Could you check a few things on this model? Use its own coordinates, in mm. A direction names the side the tool comes from. Round coordinates to 2 decimals unless told otherwise and drop trailing zeros. Write each loop counter-clockwise with the first axis right and the second up, starting at its lowest first coordinate (ties: lowest second). Pieces come first, ordered by that corner, then holes.
Autodesk Inventor part; units mm, degrees
ref_plane "YZ Plane" through (0, 0, 0) normal (1, 0, 0) x (0, 1, 0)
ref_plane "XZ Plane" through (0, 0, 0) normal (0, 1, 0) x (-1, 0, 0)
ref_plane "XY Plane" through (0, 0, 0) normal (0, 0, 1) x (1, 0, 0)
sketch "Sketch1" plane through (0, 0, 0) normal (0, 1, 0) x (-1, 0, 0)
  circle A0 centre (0, 0) radius 57
  circle A1 centre (0, 0) radius 50
  line L0 (0, -92.0258) -> (0, 121.5043)
  line L1 (123.2816, 0) -> (-123.2816, 0)
  line L2 (-50, 2) -> (50, 2)
  line L3 (50, 2) -> (50, -2)
  line L4 (50, -2) -> (-50, -2)
  line L5 (-50, -2) -> (-50, 2)
  line L6 (-50, 2) -> (50, -2) construction
  line L7 (50, 2) -> (-50, -2) construction
  line L8 (2, 50) -> (-2, 50)
  line L9 (-2, 50) -> (-2, -50)
  line L10 (-2, -50) -> (2, -50)
  line L11 (2, -50) -> (2, 50)
  line L12 (2, 50) -> (-2, -50) construction
  line L13 (-2, 50) -> (2, -50) construction
  line L14 (18.5, 91) -> (-18.5, 91)
  line L15 (-18.5, 91) -> (-18.5, 50)
  line L16 (-18.5, 50) -> (18.5, 50)
  line L17 (18.5, 50) -> (18.5, 91)
  line L18 (0, 91) -> (0, 50) construction
  line L19 (18.5, 60) -> (-18.5, 60)
  line L20 (-44.3013, -23.2679) -> (-42.3013, -26.7321)
  line L21 (-34.0513, -41.0215) -> (-52.5513, -8.9785)
  line L22 (-61.2115, -13.9785) -> (-42.7115, -46.0215)
  line L23 (-69.5583, -61.5215) -> (-34.0513, -41.0215)
  line L24 (-52.5513, -8.9785) -> (-88.0583, -29.4785)
  line L25 (-78.8083, -45.5) -> (-43.3013, -25) construction
  line L26 (-88.0583, -29.4785) -> (-69.5583, -61.5215)
  line L27 (42.3013, -26.7321) -> (44.3013, -23.2679)
  line L28 (52.5513, -8.9785) -> (34.0513, -41.0215)
  line L29 (42.7115, -46.0215) -> (61.2115, -13.9785)
  line L30 (88.0583, -29.4785) -> (52.5513, -8.9785)
  line L31 (34.0513, -41.0215) -> (69.5583, -61.5215)
  line L32 (78.8083, -45.5) -> (43.3013, -25) construction
  line L33 (69.5583, -61.5215) -> (88.0583, -29.4785)
  point P0 (2, -49.96)
  point P1 (2, -2)
  point P2 (49.96, -2)
  point P3 (-2, 49.96)
  point P4 (-2, 2)
  point P5 (-49.96, 2)
  point P6 (-2, -49.96)
  point P7 (-49.96, -2)
  point P8 (-2, -2)
  point P9 (-18.5, 53.9143)
  point P10 (-55.9411, -10.9357)
  point P11 (-37.4411, -42.9786)
  point P12 (37.4411, -42.9786)
  point P13 (55.9411, -10.9357)
  point P14 (18.5, 53.9143)
  point P15 (2, 49.96)
  point P16 (49.96, 2)
  point P17 (2, 2)
  dimension "d0" = 114
  dimension "d1" = 100
  dimension "d6" = 100
  dimension "d7" = 4
  dimension "d8" = 4
  dimension "d9" = 100
  dimension "d10" = 37
  dimension "d14" = 60
  dimension "d15" = 31
  dimension "d18" = 360
extrude "Extrusion1" add sketch "Sketch1" along normal blind 5 contours L1 L3 L2 A1 L11 L16 L17 A0 | A0 L30 L28 L27 A1 L4 L3 L1 | L17 L16 L8 L0 A0 | A0 L0 L19 L17 | L30 L29 L31 A0 | A0 L31 L28 L27 L30 | L1 L11 L2 A1 | L3 L4 A1 | A1 L4 L11 L1 | A1 L2 L3 | L0 L8 L16 L15 A0 | A0 L15 L19 L0 | L19 L0 L14 L17 | A0 L0 L10 L11 A1 L27 L28 L31 | L30 L33 L31 L29 | L11 L4 L0 L1 | L1 L0 L2 L11 | L15 L16 L9 A1 L2 L5 L1 A0 | L8 L11 A1 | L0 L2 L9 A1 | A1 L11 L2 L0 | A1 L9 L8 | L19 L15 L14 L0 | A0 L23 L21 L20 A1 L9 L10 L0 | L11 A1 L0 L4 | L1 L9 L2 L0 | L0 L4 L9 L1 | L1 L5 L4 A1 L20 L21 L24 A0 | L23 L22 L24 A0 | A0 L24 L21 L20 L23 | L10 L9 A1 | A1 L9 L4 L0 | A1 L11 L10 | L9 L4 A1 L1 | L1 A1 L2 L9 | L5 L2 A1 | A1 L4 L5 | L23 L26 L24 L22
sketch "Sketch2" plane through (0, 5, 0) normal (0, 1, 0) x (1, 0, 0)
  line L0 (-18.5, -53.9143) -> (-18.5, -91)
  line L1 (18.5, -91) -> (18.5, -53.9143)
  line L2 (-18.5, -91) -> (18.5, -91)
  line L3 (18.5, -91) -> (18.5, -60)
  line L4 (18.5, -60) -> (-18.5, -60)
  line L5 (-18.5, -60) -> (-18.5, -91)
  line L6 (-17, -61.5) -> (17, -61.5)
  line L7 (17, -61.5) -> (17, -89.5)
  line L8 (17, -89.5) -> (-17, -89.5)
  line L9 (-17, -89.5) -> (-17, -61.5)
  line L10 (88.0583, 29.4785) -> (69.5583, 61.5215)
  line L11 (69.5583, 61.5215) -> (42.7115, 46.0215)
  line L12 (42.7115, 46.0215) -> (61.2115, 13.9785)
  line L13 (61.2115, 13.9785) -> (88.0583, 29.4785)
  line L14 (61.7606, 16.0276) -> (44.7606, 45.4724)
  line L15 (44.7606, 45.4724) -> (69.0093, 59.4724)
  line L16 (69.0093, 59.4724) -> (86.0093, 30.0276)
  line L17 (86.0093, 30.0276) -> (61.7606, 16.0276)
  line L18 (-69.5583, 61.5215) -> (-88.0583, 29.4785)
  line L19 (-88.0583, 29.4785) -> (-61.2115, 13.9785)
  line L20 (-61.2115, 13.9785) -> (-42.7115, 46.0215)
  line L21 (-42.7115, 46.0215) -> (-69.5583, 61.5215)
  line L22 (-44.7606, 45.4724) -> (-61.7606, 16.0276)
  line L23 (-61.7606, 16.0276) -> (-86.0093, 30.0276)
  line L24 (-86.0093, 30.0276) -> (-69.0093, 59.4724)
  line L25 (-69.0093, 59.4724) -> (-44.7606, 45.4724)
  point P0 (0, 0)
  dimension "d22" = 31
  dimension "d23" = 1.5
  dimension "d26" = 360
extrude "Extrusion2" add sketch "Sketch2" along normal blind 46 contours L4 L1 L2 L0
sketch "Sketch4" plane through (-18.5, 0, 91) normal (0, 0, 1) x (1, 0, 0)
  line L0 (0, 51) -> (37, 51) construction
  line L1 (12.5, 51) -> (24.5, 51)
  line L2 (24.5, 51) -> (24.5, 10)
  line L3 (24.5, 10) -> (12.5, 10)
  line L4 (12.5, 10) -> (12.5, 51)
  line L5 (1.5, 5) -> (35.5, 5) construction
  line L6 (18.5, -10.2) -> (18.5, 61.2) construction
  circle A0 centre (18.5, 16) radius 6
  point P0 (18.5, 0)
  point P1 (12.5, 16)
  point P2 (24.5, 16)
  dimension "d36" = 12
  dimension "d37" = 5
  dimension "d38" = 6
extrude "Extrusion3" cut sketch "Sketch4" against normal up to next contours L1 L2 A0 L4 | A0
pattern_circular "Circular Pattern1" count 3 over 360 about axis through (0, -10, 0) along (0, 1, 0) of "Extrusion2", "Extrusion3"
sketch "Sketch5" plane through (0, 5, 0) normal (0, 1, 0) x (1, 0, 0)
  line L0 (-2, -21.5) -> (2, -21.5)
  line L1 (2, -21.5) -> (2, -17.5)
  line L2 (2, -17.5) -> (-2, -17.5)
  line L3 (-2, -17.5) -> (-2, -21.5)
  line L4 (-2, -2) -> (-2, -49.96) construction
  line L5 (2, -49.96) -> (2, -2) construction
  line L6 (-123.2816, 0) -> (123.2816, 0) construction
  line L7 (-2, 21.5) -> (2, 21.5)
  line L8 (2, 21.5) -> (2, 17.5)
  line L9 (2, 17.5) -> (-2, 17.5)
  line L10 (-2, 17.5) -> (-2, 21.5)
  arc A0 (-49.96, -2) -> (-2, -49.96) centre (0, 0) ccw construction
  arc A1 (-2, 49.96) -> (-49.96, 2) centre (0, 0) ccw construction
  circle A2 centre (0, 0) radius 50 construction
  line L11 (-54, 6) -> (-50, 6)
  line L12 (-50, 6) -> (-50, -6)
  line L13 (-50, -6) -> (-54, -6)
  line L14 (-54, -6) -> (-54, 6)
  line L15 (-54, 0) -> (-50, 0) construction
  line L16 (0, 92.0258) -> (0, -121.5043) construction
  line L17 (54, 6) -> (50, 6)
  line L18 (50, 6) -> (50, -6)
  line L19 (50, -6) -> (54, -6)
  line L20 (54, -6) -> (54, 6)
  line L21 (54, 0) -> (50, 0) construction
  point P0 (49.96, -2)
  point P1 (49.96, 2)
  dimension "d41" = 17.5
  dimension "d42" = 4
  dimension "d43" = 12
extrude "Extrusion4" add sketch "Sketch5" along normal blind 10
equation "\"d38\" = 0.5 * d36"
properties part number "bottom"
Q1. We'd pull the mould along X, two halves only. Please class faces 1 (the flat face through (52, 10, 6)), 2 (the flat face through (-74.823, 27.678, -21.837)), 3 (the flat face through (71.775, 2.465, -20.077)), 4 (the flat face through (-26, 2, -2)): pulls with the +X half, pulls with the -X half, needs draft (parallel to the pull), parting line crosses it, or undercut.
Q2. On a 3-axis mill with a long thin cutter (end or side, diameter ignored), from which of +Z, -Z, +X, -X, +Y, -Y can I reach the whole of each face in a straight line? I mean faces 5 (the cylindrical face through (-34.984, 2.465, 35.722)), 6 (the flat face through (-7, 28, 89.5)), 7 (the flat face through (52, 10, -6)). Say none if no direction works.
Q3. Imagine slicing it at C-C, the plane z = 47.5. Write out the boundary of the cut face in (x, y), then the cut area to 3 significant figures.
Q4. If I drill on L1, parallel to Z at x = -6, y = 9; L2, parallel to X at y = 7, z = 82.5; L3, parallel to X at y = 2, z = -23.5, over which ranges is the centre line in solid material (lowest first)?
Q5. Imagine slicing it at B-B, the plane y = 18. Count the separate pieces of the cut face and the enclosed holes in it, then the cut area to 3 significant figures.
Q6. I'm going to push flat-ended pins straight in: pin 1 Ø1.2 at (x, y) = (-0.5, 9) entering from -Z; pin 2 Ø10 at (y, z) = (10.5, 19) entering from +X; pin 3 Ø8 at (y, z) = (10.5, -33.5) entering from -X. Where does each tip first touch, or does it pass through?
Results found:
1. face 1: needs draft
1. face 2: pulls with the -X half
1. face 3: pulls with the +X half
1. face 4: undercut
2. face 5: +Y, -Y
2. face 6: +Y
2. face 7: +X, -X, +Y
3. outline: (-31.51, 0) - (-15.61, 0) - (-15.61, 5) - (-31.51, 5) - close; (-2, 0) - (2, 0) - (2, 5) - (-2, 5) - close; (15.61, 0) - (31.51, 0) - (31.51, 5) - (15.61, 5) - close
3. area: 179 mm2
4. L1: z = 60 to 61.5, 89.5 to 91
4. L2: x = -18.5 to -17, 17 to 18.5
4. L3: x = -77.7 to -44.13, -2 to 2, 44.13 to 77.7
5. separate pieces: 3
5. enclosed holes: 0
5. area: 531 mm2
6. pin 1: stops at z = -21.5
6. pin 2: stops at x = 2
6. pin 3: stops at x = -88.05
